Design review of the part built by this model. Coordinates are the model's own, in mm. Coordinates: 2 decimals unless noted, no trailing zeros. Loops run counter-clockwise (first coordinate to the right, second up) from the corner with the lowest first, then second, coordinate; pieces in that order, holes last. Notation, with made-up numbers: M -19,12.5 L 1,12.5 A8 cw 1,24.5 Z; hole C 83.25,12.25 d2. An arc over 180 degrees is marked long. One line per item, written item: value.
```python
from build123d import *

# Parameters (mm, degrees)
EXTRUDE_1_DEPTH     = 2.2
SKETCH_3_R          = 4.365
EXTRUDE_2_DEPTH     = 1.4
SKETCH_4_R          = 2.085
CUT_EXTRUDE_1_DEPTH = 9.837280407
EXTRUDE_START       = -0.2
SKETCH_5_R          = 2.085
SKETCH_5_R_2        = 1.96
EXTRUDE_3_DEPTH     = 1.2
FILLET_1_R          = 0.575


with BuildPart() as part:
    # 草图1 → 凸台-拉伸1 (new, symmetric)
    with BuildSketch(Plane(origin=(0, 0, 0), x_dir=(1, 0, 0), z_dir=(0, 1, 0))):
        Polygon((5.04026785, 0), (2.520133925, 4.365), (-2.520133925, 4.365), (-5.04026785, 0), (-2.520133925, -4.365), (2.520133925, -4.365), align=None)
    extrude(amount=EXTRUDE_1_DEPTH, both=True)

    # 草图3 → 凸台-拉伸2 (add)
    with BuildSketch(Plane(origin=(0, 2.2, 0), x_dir=(1, 0, 0), z_dir=(0, 1, 0))):
        with Locations(Location((0, 0, 0), (0, 0, 270))):
            Circle(SKETCH_3_R)
    extrude(amount=EXTRUDE_2_DEPTH)

    # 草图4 → 切除-拉伸1 (cut, through all)
    with BuildSketch(Plane(origin=(0, 3.6, 0), x_dir=(1, 0, 0), z_dir=(0, 1, 0))):
        with Locations(Location((0, 0, 0), (0, 0, 270))):
            Circle(SKETCH_4_R)
    extrude(amount=-CUT_EXTRUDE_1_DEPTH, mode=Mode.SUBTRACT)

    # 草图5 → 凸台-拉伸3 (add)
    with BuildSketch(Plane(origin=(0, 3.6, 0), x_dir=(1, 0, 0), z_dir=(0, 1, 0)).offset(EXTRUDE_START)):
        with Locations(Location((0, 0, 0), (0, 0, 270))):
            Circle(SKETCH_5_R)
        with Locations(Location((0, 0, 0), (0, 0, 270))):
            Circle(SKETCH_5_R_2, mode=Mode.SUBTRACT)
    extrude(amount=-EXTRUDE_3_DEPTH)

    # 圆角1
    # the kernel refuses this fillet: 0.575 mm, written as the material it takes off along each edge
    with BuildSketch(Plane(origin=(0, 3.6, 0), x_dir=(0, 0, 1), z_dir=(-1, 0, 0))) as fillet_1_piece_1:
        with BuildLine():
            CenterArc((4.365 - FILLET_1_R, -FILLET_1_R), FILLET_1_R, 0, 90)
            Line((4.365 - FILLET_1_R, 0), (4.365 - FILLET_1_R, FILLET_1_R * 0.02))
            Line((4.365 - FILLET_1_R, FILLET_1_R * 0.02), (4.365 + FILLET_1_R * 0.02, FILLET_1_R * 0.02))
            Line((4.365 + FILLET_1_R * 0.02, FILLET_1_R * 0.02), (4.365 + FILLET_1_R * 0.02, -FILLET_1_R))
            Line((4.365 + FILLET_1_R * 0.02, -FILLET_1_R), (4.365, -FILLET_1_R))
        make_face()
    revolve(axis=Axis((0, 3.6, 0), (0, 1, 0)), mode=Mode.SUBTRACT)
    with BuildSketch(Plane(origin=(0, 3.6, 0), x_dir=(0, 0, 1), z_dir=(-1, 0, 0))) as fillet_1_piece_2:
        with BuildLine():
            CenterArc((2.520889894, -0.575), FILLET_1_R, 90, 49.294293169)
            Line((2.085, -0.2), (2.076282202, -0.1925))
            ThreePointArc((2.076282202, -0.1925), (2.0735, -0.1), (2.0735, 0))
            Line((2.0735, 0), (2.085, 0.0115))
            Line((2.085, 0.0115), (2.520889894, 0.0115))
            Line((2.520889894, 0.0115), (2.520889894, 0))
        make_face()
    revolve(axis=Axis((0, 3.6, 0), (0, 1, 0)), mode=Mode.SUBTRACT)

    # 草图6 → 切除-旋转1 (revolve, cut)
    with BuildSketch(Plane.XY):
        Polygon((-5.04026785, 2.2), (-5.04026785, 1.52473215), (-4.365, 2.2), align=None)
        Polygon((-5.04026785, -2.2), (-5.04026785, -1.52473215), (-4.365, -2.2), align=None)
    revolve(axis=Axis((0, -1000, 0), (0, 1, 0)), mode=Mode.SUBTRACT)


solid = part.part
```
(1) We need section C-C on y = 2.8. State the section outline as (x, z) points (3 decimals).
Reply:
outline: C 0,0 d8.73; hole C 0,0 d3.92
(2) Mouldability with a two-part tool opening along X and no side actions: class faces 1 (the flat face through (3.763, 0.031, 2.213)), 2 (the cylindrical face through (-0.75, 2.81, 1.81)), 3 (the cylindrical face through (4.328, 2.607, -0.568)) as released by +X, released by -X, zero draft, split by the parting line, or undercut.
Reply:
face 1: released by +X
face 2: undercut
face 3: split by the parting line
(3) To check wall thickness, follow line 1 along X through (y, z) = (3.05, 0); line 2 along Z through (x, y) = (1.25, 1.15) (3 decimals); line 3 along X through (y, z) = (1.25, 1.5). State the ranges of each line that lie inside material, in increasing order. Write a range as [from, to].
Reply:
line 1: x = [-4.36, -1.96], [1.96, 4.36]
line 2: z = [-4.365, -1.669], [1.669, 4.365]
line 3: x = [-4.17, -1.45], [1.45, 4.17]
(4) We need section B-B on y = -1.75. State the section outline as (x, z) points (3 decimals).
Reply:
outline: M -4.796,-0.422 L -2.764,-3.943 A4.815 ccw -2.032,-4.365 L 2.032,-4.365 A4.815 ccw 2.764,-3.943 L 4.796,-0.422 A4.815 ccw 4.796,0.422 L 2.764,3.943 A4.815 ccw 2.032,4.365 L -2.032,4.365 A4.815 ccw -2.764,3.943 L -4.796,0.422 A4.815 ccw Z; hole C 0,0 d4.17
(5) We need section A-A on y = 1.2. State the section outline as (x, z) points (3 decimals), then the cut area to 3 significant figures.
Reply:
outline: M -5.04,0 L -2.52,-4.365 L 2.52,-4.365 L 5.04,0 L 2.52,4.365 L -2.52,4.365 Z; hole C 0,0 d4.17
area: 52.3 mm2
